CAD build for the part. Positions are in the model's coordinates, mm. Face numbers are marked on the shaded views. A direction names the side the tool comes from. Give positions to 0.01 mm unless a question says otherwise; leave off trailing zeros. Order: outer loops, then holes, each group sorted by start corner. A loop starts at its lowest first (then second) coordinate and runs counter-clockwise, first axis right, second up.
Item 1: Flat gauge pins, fed straight in: P1, Ø8, axis at x = -82.5, y = 10, coming from the +Z side; P2, Ø1.5, axis at x = 13.5, y = 57.5, coming from the -Z side; P3, Ø12, axis at x = -59, y = 36.5, coming from the +Z side; P4, Ø23.5, axis at y = 24, z = -134.5, coming from the +X side. Where does each tip first touch, or does it go through?
Item 2: Band-saw the part on C-C on z = -81.5. Give the cut face in (x, y).
Item 3: Two-plate mould, pull along X, no slides. Class the marked faces 3, 4 and 5: released by +X, released by -X, zero draft, split by the parting line, or undercut.
Item 4: Band-saw the part on A-A on x = 0. Give the cut face in (y, z), plus the area to 3 significant figures.
Item 5: Which spindle directions (+Z, -Z, +X, -X, +Y, -Y) get a long thin tool onto all of the face, cutting with end or side? Do the marked faces 1 and 2. Say none if no direction does.
Item 6: Band-saw the part on B-B on z = -63. Give the cut face in (x, y).
Item 7: Band-saw the part on D-D on y = 59. Count the separate pieces of the cut face and the enclosed holes in it, plus the area to 3 significant figures.
Item 8: Wall check: L1, parallel to X at y = 16, z = -149; L2, parallel to X at y = 16, z = -136; L3, parallel to Y at x = 0, z = -140. Give the ranges that are in metal, low to high.
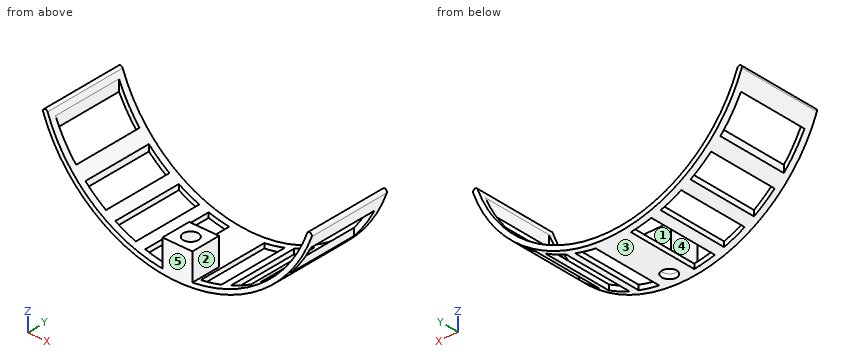
```python
from build123d import *

# Parameters (mm, degrees)
BOSS_EXTRUDE1_DEPTH = 90
BOSS_EXTRUDE2_REACH = 155
SKETCH2_W           = 32
SKETCH2_H           = 32
SKETCH2_R           = 8
SKETCH3_R           = 8
CUT_EXTRUDE1_DEPTH  = 210
SKETCH4_W           = 32
SKETCH4_H           = 118
CUT_EXTRUDE2_DEPTH  = 210
SKETCH5_W           = 22
SKETCH5_H           = 76
CUT_EXTRUDE4_DEPTH  = 210


with BuildPart() as part:
    # Sketch1 → Boss-Extrude1 (new body)
    with BuildSketch(Plane(origin=(0, 0, 0), x_dir=(1, 0, 0), z_dir=(0, 1, 0))):
        with BuildLine():
            ThreePointArc((139.074507876, 50.618981212), (0, 148), (-139.074507876, 50.618981212))
            ThreePointArc((-139.074507876, 50.618981212), (-142.278789787, 49.124800019), (-143.77297098, 52.329081929))
            ThreePointArc((-143.77297098, 52.329081929), (0, 153), (143.77297098, 52.329081929))
            ThreePointArc((143.77297098, 52.329081929), (142.278789787, 49.124800019), (139.074507876, 50.618981212))
        make_face()
    extrude(amount=BOSS_EXTRUDE1_DEPTH)

    # Sketch2 → Boss-Extrude2 (add, up to next)
    with BuildSketch(Plane.XY, mode=Mode.PRIVATE) as boss_extrude2_sk1:
        with Locations((0, 16)):
            Rectangle(SKETCH2_W, SKETCH2_H)
        with Locations((0, 16)):
            Circle(SKETCH2_R, mode=Mode.SUBTRACT)
    boss_extrude2_tool1 = extrude(boss_extrude2_sk1.sketch, amount=-BOSS_EXTRUDE2_REACH, mode=Mode.PRIVATE) - part.part
    add(boss_extrude2_tool1.solids().sort_by_distance((0, 0.452548, 0))[0])

    # Sketch3 → Cut-Extrude1 (cut)
    with BuildSketch(Plane.XY):
        with Locations((0, 16)):
            Circle(SKETCH3_R)
    extrude(amount=-CUT_EXTRUDE1_DEPTH, mode=Mode.SUBTRACT)

    # Sketch4 → Cut-Extrude2 (cut)
    with BuildSketch(Plane(origin=(0, 32, 0), x_dir=(1, 0, 0), z_dir=(0, 1, 0))):
        with Locations((0, 59)):
            Rectangle(SKETCH4_W, SKETCH4_H)
    extrude(amount=-CUT_EXTRUDE2_DEPTH, mode=Mode.SUBTRACT)

    # Sketch5 → Cut-Extrude4 (cut)
    with BuildSketch(Plane(origin=(0, 0, -153), x_dir=(-1, 0, 0), z_dir=(0, 0, -1))):
        with Locations((-125.77297098, 45)):
            Rectangle(SKETCH5_W, SKETCH5_H)
        with Locations((-93.77297098, 45)):
            Rectangle(SKETCH5_W, SKETCH5_H)
        with Locations((-61.77297098, 45)):
            Rectangle(SKETCH5_W, SKETCH5_H)
        with Locations((29.77297098, 45)):
            Rectangle(SKETCH5_W, SKETCH5_H)
        with Locations((61.77297098, 45)):
            Rectangle(SKETCH5_W, SKETCH5_H)
        with Locations((93.77297098, 45)):
            Rectangle(SKETCH5_W, SKETCH5_H)
        with Locations((125.77297098, 45)):
            Rectangle(SKETCH5_W, SKETCH5_H)
        with Locations((-29.77297098, 45)):
            Rectangle(SKETCH5_W, SKETCH5_H)
    extrude(amount=-CUT_EXTRUDE4_DEPTH, mode=Mode.SUBTRACT)


solid = part.part
```
The answers:
1. P1: stops at z = -121.05
1. P2: stops at z = -152.47
1. P3: passes through
1. P4: stops at x = 82.77
2. outline: (-129.49, 0) - (-123.54, 0) - (-123.54, 7) - (-129.49, 7) - close; (-129.49, 83) - (-123.54, 83) - (-123.54, 90) - (-129.49, 90) - close; (123.54, 0) - (129.49, 0) - (129.49, 7) - (123.54, 7) - close; (123.54, 83) - (129.49, 83) - (129.49, 90) - (123.54, 90) - close
3. face 3: split by the parting line
3. face 4: undercut
3. face 5: zero draft
4. outline: (0, -153) - (8, -153) - (8, -118) - (0, -118) - close; (24, -153) - (90, -153) - (90, -148) - (32, -148) - (32, -118) - (24, -118) - close
4. area: 850 mm2
5. face 1: +Z, +Y
5. face 2: +Z, +Y, -Y
6. outline: (-139.43, 0) - (-133.92, 0) - (-133.92, 7) - (-136.77, 7) - (-136.77, 83) - (-133.92, 83) - (-133.92, 90) - (-139.43, 90) - close; (133.92, 0) - (139.43, 0) - (139.43, 90) - (133.92, 90) - (133.92, 83) - (136.77, 83) - (136.77, 7) - (133.92, 7) - close
7. separate pieces: 9
7. enclosed holes: 0
7. area: 698 mm2
8. L1: x = -18.77 to -8, 8 to 18.77
8. L2: x = -16 to -8, 8 to 16
8. L3: y = 0 to 8, 24 to 32
